from build123d import *

# Parameters (mm, degrees)
BASPROSKE_W         = 9.525
BASPROSKE_H         = 11.1125
TOOTHCUT_DEPTH      = 19.376641083
TEETHCUTS_COUNT     = 12
TEETHCUTS_ANGLE     = 330
BORSKE_R            = 3.175
BORE_DEPTH          = 50.8000508
BOSS_EXTRUDE1_START = -25.4
SKETCH2_R           = 7.539355
BOSS_EXTRUDE1_DEPTH = 25.4
CUT_EXTRUDE1_DEPTH  = 20
SKETCH5_R           = 1.905
CUT_EXTRUDE2_DEPTH  = 24.605363577
SKETCH6_R           = 12.7
SKETCH6_R_2         = 5.7785
CUT_EXTRUDE3_DEPTH  = 15.875


with BuildPart() as part:
    # BasProSke → Base-Revolve (revolve)
    with BuildSketch(Plane(origin=(0, 0, 0), x_dir=(1, 0, 0), z_dir=(0, 1, 0)), mode=Mode.PRIVATE) as base_revolve_sk:
        with Locations((4.7625, 5.55625)):
            Rectangle(BASPROSKE_W, BASPROSKE_H)
    revolve(base_revolve_sk.sketch.rotate(Axis((-10, 0, 0), (1, 0, 0)), 180), axis=Axis((-10, 0, 0), (1, 0, 0)))

    # TooCutSke → ToothCut (cut, through all)
    with BuildSketch(Plane(origin=(0, 0, 0), x_dir=(0, 0, -1), z_dir=(1, 0, 0))):
        with BuildLine():
            ThreePointArc((1.026937745, 7.469087808), (0, 7.539355), (-1.026937745, 7.469087808))
            ThreePointArc((-1.026937745, 7.469087808), (-1.30857978, 9.35080814), (-2.465050847, 10.861691431))
            ThreePointArc((-2.465050847, 10.861691431), (0, 11.1379), (2.465050847, 10.861691431))
            ThreePointArc((2.465050847, 10.861691431), (1.30857978, 9.35080814), (1.026937745, 7.469087808))
        make_face()
    toothcut = extrude(amount=TOOTHCUT_DEPTH, mode=Mode.SUBTRACT)

    # TeethCuts: ToothCut ×12 about axis
    teethcuts_axis = Axis((-10, 0, 0), (1, 0, 0))
    for i in range(1, TEETHCUTS_COUNT):
        add(toothcut.rotate(teethcuts_axis, i * TEETHCUTS_ANGLE / (TEETHCUTS_COUNT - 1)), mode=Mode.SUBTRACT)

    # BorSke → Bore (cut, symmetric)
    with BuildSketch(Plane(origin=(0, 0, 0), x_dir=(0, 0, -1), z_dir=(1, 0, 0))):
        with Locations(Location((0, 0, 0), (0, 0, 180))):
            Circle(BORSKE_R)
    extrude(amount=BORE_DEPTH, both=True, mode=Mode.SUBTRACT)

    # Sketch2 → Boss-Extrude1 (add)
    with BuildSketch(Plane(origin=(9.525, 0, 0), x_dir=(0, 0, -1), z_dir=(1, 0, 0)).offset(BOSS_EXTRUDE1_START)):
        with Locations(Location((0, 0, 0), (0, 0, 172.171388978))):
            Circle(SKETCH2_R)
    extrude(amount=BOSS_EXTRUDE1_DEPTH)

    # Sketch3 → Cut-Extrude1 (cut)
    with BuildSketch(Plane.ZY.offset(15.875)):
        with BuildLine():
            Line((-1.778, 2.8575), (1.778, 2.8575))
            ThreePointArc((1.778, 2.8575), (0, -3.3655), (-1.778, 2.8575))
        make_face()
    extrude(amount=-CUT_EXTRUDE1_DEPTH, mode=Mode.SUBTRACT)

    # Sketch5 → Cut-Extrude2 (cut, through all)
    with BuildSketch(Plane.XZ.offset(-2.8575)):
        with Locations(Location((-12.065, 0, 0), (0, 0, 270))):
            Circle(SKETCH5_R)
    extrude(amount=-CUT_EXTRUDE2_DEPTH, mode=Mode.SUBTRACT)

    # Sketch6 → Cut-Extrude3 (cut)
    with BuildSketch(Plane.ZY.offset(15.875)):
        Circle(SKETCH6_R)
        Circle(SKETCH6_R_2, mode=Mode.SUBTRACT)
    extrude(amount=-CUT_EXTRUDE3_DEPTH, mode=Mode.SUBTRACT)


solid = part.part
For this review, take the finished solid that the model builds, in its own axes (mm). Round coordinates to 2 decimals unless told otherwise and drop trailing zeros. Loops run counter-clockwise (first coordinate to the right, second up) from the corner with the lowest first, then second, coordinate; pieces in that order, holes last. Notation, with made-up numbers: (26, 83.5) - (32, 83.5) arc R21 ccw to (32, 115.5) - close; hole circle Ø8 at (-11.5, 59.25). An arc over 180 degrees is marked (long way). One line per question, with ' | ' between items.
Q1. For pin 1 (4 mm diameter, centred on x = 0, y = 3, fed in from -Z); pin 2 (3 mm diameter, centred on y = 0.5, z = 1.5, fed in from -X) (3 decimals); pin 3 (1.1 mm diameter, centred on x = -7, z = 0.5, fed in from -Y); pin 4 (4 mm diameter, centred on x = 3.5, z = -8, fed in from -Y), all flat-tipped, find the tip position at first contact; note any pin that passes through.
Taken from the geometry:
pin 1: stops at z = -10.84 | pin 2: stops at x = 4.125 | pin 3: stops at y = -5.78 | pin 4: stops at y = -8.17
Q2. Take a section at D-D (x = -5). Give the boundary of the cut face in (y, z), and give its area (3 significant figures).
Taken from the geometry:
outline: circle Ø11.56 at (0, 0); hole (2.86, -1.78) - (2.86, 1.78) arc R3.37 ccw (long way) to start | area: 70.5 mm²
Q3. Take a section at B-B (y = 0). Give the boundary of the cut face in (x, z) (1 decimal).
Taken from the geometry:
outline: (-15.9, -5.8) - (0, -5.8) - (0, -7.5) - (9.5, -7.5) - (9.5, 7.5) - (0, 7.5) - (0, 5.8) - (-15.9, 5.8) - (-15.9, 3.4) - (4.1, 3.4) - (4.1, -3.4) - (-15.9, -3.4) - close
Q4. Take a section at C-C (y = -8.5). Give the boundary of the cut face in (x, z) (3 decimals).
Taken from the geometry:
outline: (0, -3.502) - (9.525, -3.502) - (9.525, -1.06) - (0, -1.06) - close; (0, 1.06) - (9.525, 1.06) - (9.525, 3.502) - (0, 3.502) - close
Q5. For line 1 along Y through (x, z) = (-3, 0); line 2 along X through (y, z) = (4.3, 0) (3 decimals); line 3 along X through (y, z) = (-3, 9.75) (3 decimals), list the stretches that pass through material, from the lowest coordinate up. Write a range as [from, to].
Taken from the geometry:
line 1: y = [-5.78, -3.37], [2.86, 5.78] | line 2: x = [-15.875, -13.97], [-10.16, 9.525] | line 3: x = [0, 9.525]
Q6. The part is to be moulded in two halves that separate along Z. For faces 1 (the cylindrical face through (-8.05, -5.64, -1.25)), 2 (the cylindrical face through (4.696, 7.418, 5.774)), 3 (the cylindrical face through (4.829, 10.732, -2.882)), say which applies: released by +Z, released by -Z, zero draft, split by the parting line, or undercut.
Taken from the geometry:
face 1: split by the parting line | face 2: undercut | face 3: released by -Z
Q7. Take a section at A-A (z = 0). Give the boundary of the cut face in (x, y) (1 decimal).
Taken from the geometry:
outline: (-15.9, -5.8) - (0, -5.8) - (0, -7.5) - (9.5, -7.5) - (9.5, 7.5) - (0, 7.5) - (0, 5.8) - (-10.2, 5.8) - (-10.2, 2.9) - (4.1, 2.9) - (4.1, -3.4) - (-15.9, -3.4) - close; (-15.9, 2.9) - (-14, 2.9) - (-14, 5.8) - (-15.9, 5.8) - close
